Here's how the part is built. I have some questions about the finished solid (model axes, mm). A direction names the side the tool comes from. Coordinates: 2 decimals unless noted, no trailing zeros. Loops run counter-clockwise (first coordinate to the right, second up) from the corner with the lowest first, then second, coordinate; pieces in that order, holes last. Notation, with made-up numbers: (60.5, 31.25) -> (98.5, 31.25) arc R23 cw to (98.5, 47.25) -> close; hole circle Ø6 at (74, 73). An arc over 180 degrees is marked (long way). Answer as a JSON object with one key per item and string values. Group by question number.
Q1. I'm going to push flat-ended pins straight in: pin 1 (12 mm diameter, centred on x = -62.5, z = -59, fed in from +Y); pin 2 (3 mm diameter, centred on x = -132.25, y = 126.75, fed in from -Z); pin 3 (12 mm diameter, centred on x = -136, y = 125, fed in from +Z); pin 4 (3 mm diameter, centred on y = 130.5, z = -85.5, fed in from -X). Where does each tip first touch, or does it pass through?
Q2. I want a section at B-B on x = -138.75. Write out the boundary of the cut face in (y, z), then the cut area to 4 significant figures.
Q3. I want a section at D-D on z = -32.5. Write out the boundary of the cut face in (x, y).
Q4. Thinking about a two-plate mould opening in X: for faces 1 (the flat face through (-136, 128, -90)), 2 (the cylindrical face through (-62.2, 115.23, -90.14)), 3 (the flat face through (-50.5, 105, -62)), which applies, released by +X, released by -X, zero draft, split by the parting line, or undercut?
Q5. I want a section at A-A on y = 126.75. Write out the boundary of the cut face in (x, z).
Q6. I need wall thicknesses on line 1 (Y direction, x = -132, z = -94); line 2 (X direction, y = 135, z = -88.25); line 3 (Y direction, x = -58.5, z = -26). Which ranges of each line are inside material? Lowest first, please.
Q7. I want a section at C-C on x = -127. Write out the boundary of the cut face in (y, z), then the cut area to 3 significant figures.
Q8. On a 3-axis mill with a long thin cutter (end or side, diameter ignored), from which of +Z, -Z, +X, -X, +Y, -Y can I reach the whole of each face in a straight line? I mean faces 4 (the flat face through (-85, 128, -80)), 5 (the flat face through (-90, 145, -90)), 6 (the flat face through (-120.5, 128, -85)). Say none if no direction works.
Autodesk Inventor part; units mm, degrees
ref_plane "YZ Plane" through (0, 0, 0) normal (1, 0, 0) x (0, 1, 0)
ref_plane "XZ Plane" through (0, 0, 0) normal (0, 1, 0) x (-1, 0, 0)
ref_plane "XY Plane" through (0, 0, 0) normal (0, 0, 1) x (1, 0, 0)
sketch "Boceto2" plane through (0, 0, 0) normal (0, 1, 0) x (-1, 0, 0)
  line L0 (7.5, 100) -> (-7.5, 100)
  line L1 (-7.5, 100) -> (-7.5, -100)
  line L2 (-7.5, -100) -> (7.5, -100)
  line L3 (7.5, -100) -> (7.5, 100)
  line L4 (7.5, 100) -> (-7.5, -100) construction
  line L5 (-7.5, 100) -> (7.5, -100) construction
  point P0 (0, 0)
  dimension "d7" = 15
  dimension "d8" = 200
extrude "Extrusión1" add sketch "Boceto2" along normal blind 10
sketch "Boceto3" plane through (0, 10, 0) normal (0, 1, 0) x (1, 0, 0)
  circle A0 centre (3.25, 58.25) radius 1.75
  line L0 (5, 50) -> (-5, 50)
  line L1 (-5, 50) -> (-5, 60)
  line L2 (-5, 60) -> (5, 60)
  line L3 (5, 60) -> (5, 50)
  line L4 (5, 50) -> (-5, 60) construction
  line L5 (-5, 50) -> (5, 60) construction
  circle A1 centre (-3.25, 51.75) radius 1.75
  line L6 (7.5, 100) -> (-7.5, 100)
  line L7 (-7.5, 0) -> (3.408, 0)
  line L8 (5, -60) -> (5, -50)
  line L9 (-5, -60) -> (5, -60)
  line L10 (5, -50) -> (-5, -50)
  line L11 (-5, -50) -> (-5, -60)
  line L12 (-5, -50) -> (5, -60) construction
  circle A2 centre (-3.25, -51.75) radius 1.75
  line L13 (5, -50) -> (-5, -60) construction
  circle A3 centre (3.25, -58.25) radius 1.75
  line L14 (-7.5, -100) -> (7.5, -100)
  point P0 (0, 0)
  point P1 (-5, 55)
  point P2 (0, 100)
  point P3 (-5, -55)
  dimension "d11" = 3.5
  dimension "d12" = 1.75
  dimension "d13" = 1.75
  dimension "d14" = 1.75
  dimension "d15" = 1.75
  dimension "d16" = 10
  dimension "d17" = 10
  dimension "d19" = 40
  dimension "d81" = 40
hole "Agujero1" at (3.25, 10, 58.25) at (-3.25, 10, 51.75) at (3.25, 10, -58.25) at (-3.25, 10, -51.75) direction (0, -1, 0) diameter 3.5 end through all
sketch "Boceto4" plane through (0, 10, 0) normal (0, 1, 0) x (1, 0, 0)
  line L0 (-7.5, 100) -> (-7.5, -100)
  line L1 (-7.5, -100) -> (7.5, -100)
  line L2 (7.5, -100) -> (7.5, -80)
  line L3 (7.5, -80) -> (-7.5, -80)
  line L4 (-7.5, -80) -> (-7.5, -100)
  line L5 (-7.5, 0) -> (1.0116, 0)
  line L6 (-7.5, -100) -> (-7.5, 100)
  line L7 (-7.5, 100) -> (7.5, 100)
  line L8 (7.5, 100) -> (7.5, 80)
  line L9 (7.5, 80) -> (-7.5, 80)
  line L10 (-7.5, 80) -> (-7.5, 100)
  point P0 (0, 0)
  point P1 (-7.5, -80)
  point P2 (-7.5, 80)
  dimension "d27" = 15
  dimension "d28" = 20
extrude "Extrusión2" add sketch "Boceto4" along normal blind 80
sketch "Boceto5" plane through (0, 90, 0) normal (0, 1, 0) x (1, 0, 0)
  line L0 (-7.5, -100) -> (7.5, -100)
  line L1 (-7.5, -100) -> (49.5, -100)
  line L2 (49.5, -100) -> (49.5, 100)
  line L3 (49.5, 100) -> (-7.5, 100)
  line L4 (-7.5, 100) -> (-7.5, -100)
  line L5 (49.5, -100) -> (-150.5, -100)
  line L6 (-150.5, -100) -> (-150.5, 100)
  line L7 (-150.5, 100) -> (49.5, 100)
  line L8 (49.5, 100) -> (49.5, -100)
  point P0 (0, 0)
  point P1 (-7.5, 100)
  dimension "d31" = 57
  dimension "d32" = 200
  dimension "d75" = 200
extrude "Extrusión3" add sketch "Boceto5" along normal blind 110
sketch "Boceto6" plane through (0, 200, 0) normal (0, 1, 0) x (1, 0, 0)
  line L0 (49.5, 100) -> (7.5, 100)
  line L1 (49.5, 100) -> (29.5, 100)
  line L2 (29.5, 100) -> (29.5, 80)
  line L3 (7.5, -100) -> (49.5, -100)
  line L4 (28.5, -100) -> (28.5, -80)
  line L5 (-150.5, 100) -> (-150.5, -100)
  line L6 (29.5, 80) -> (-150.5, 80)
  line L7 (-150.5, 80) -> (-150.5, -80)
  line L8 (-150.5, -80) -> (29.5, -80)
  line L9 (29.5, -80) -> (29.5, 80)
  line L10 (-150.5, -100) -> (49.5, -100)
  point P0 (7.5, 80)
  point P1 (-50.5, -100)
  dimension "d36" = 20
  dimension "d37" = 20
  dimension "d38" = 20
  dimension "d77" = 20
extrude "Extrusión4" cut sketch "Boceto6" against normal blind 90 contours L8 L5 L6 L9
sketch "Boceto7" plane through (-150.5, 90, -100) normal (-1, 0, 0) x (0, 0, 1)
  line L0 (0, 110) -> (20, 110)
  line L1 (20, 110) -> (10, 110)
  line L2 (10, 110) -> (10, 20)
  line L3 (10, 20) -> (20, 20)
  line L4 (20, 20) -> (20, 110)
  line L5 (180, 110) -> (180, 20)
  line L6 (180, 110) -> (190, 110)
  line L7 (190, 110) -> (190, 20)
  line L8 (190, 20) -> (180, 20)
  line L9 (180, 20) -> (180, 110)
  line L10 (200, 0) -> (200, 110)
  line L11 (0, 0) -> (0, 110)
  line L12 (0, 110) -> (10, 110)
  line L13 (10, 110) -> (10, 20)
  line L14 (10, 20) -> (0, 20)
  line L15 (0, 20) -> (0, 110)
  line L16 (200, 110) -> (0, 110)
  line L17 (200, 110) -> (190, 110)
  line L18 (190, 110) -> (190, 20)
  line L19 (190, 20) -> (200, 20)
  line L20 (200, 20) -> (200, 110)
  point P0 (100, -90)
  dimension "d63" = 10
  dimension "d65" = 10
  dimension "d76" = 10
extrude "Extrusión5" cut sketch "Boceto7" against normal blind 30 contours L6 L7 L8 L5 | L0 L4 L3 L2
sketch "Boceto8" plane through (-7.5, 0, 100) normal (0, 0, 1) x (1, 0, 0)
  line L0 (-113, 110) -> (-113, 200)
  line L1 (-113, 200) -> (-113, 110)
  circle A0 centre (-124.75, 183.25) radius 1.75
  line L2 (-123, 175) -> (-133, 175)
  line L3 (-133, 175) -> (-133, 185)
  line L4 (-133, 185) -> (-123, 185)
  line L5 (-123, 185) -> (-123, 175)
  line L6 (-123, 175) -> (-133, 185) construction
  line L7 (-133, 175) -> (-123, 185) construction
  circle A1 centre (-131.25, 176.75) radius 1.75
  line L8 (-143, 200) -> (57, 200)
  line L9 (-143, 90) -> (-143, 200)
  line L10 (-113, 155) -> (-128, 155)
  line L11 (-123, 125) -> (-123, 135)
  line L12 (-133, 125) -> (-123, 125)
  line L13 (-123, 135) -> (-133, 125) construction
  line L14 (-123, 135) -> (-133, 135)
  line L15 (-133, 135) -> (-123, 125) construction
  circle A2 centre (-131.25, 133.25) radius 1.75
  line L16 (-133, 135) -> (-133, 125)
  circle A3 centre (-124.75, 126.75) radius 1.75
  line L17 (-143, 110) -> (-113, 110)
  point P0 (7.5, 0)
  point P1 (-133, 180)
  point P2 (-123, 180)
  point P3 (-133, 130)
  point P4 (-123, 130)
  dimension "d45" = 3.5
  dimension "d46" = 1.75
  dimension "d47" = 1.75
  dimension "d48" = 1.75
  dimension "d49" = 1.75
  dimension "d50" = 10
  dimension "d51" = 10
  dimension "d52" = 15
  dimension "d53" = 10
  dimension "d54" = 10
  dimension "d55" = 15
hole "Agujero2" at (-132.25, 183.25, 100) at (-138.75, 176.75, 100) at (-138.75, 133.25, 100) at (-132.25, 126.75, 100) direction (0, 0, -1) diameter 3.5 end through all
ref_plane "Plano de trabajo1" through (-150.5, 90, 100) normal (0, -1, 0) x (1, 0, 0)
split "Dividir1" plane through (-150.5, 90, 100) removes the side toward (0, -1, 0)
ref_plane "Plano de trabajo2" through (49.5, 90, 0) normal (0, 0, -1) x (-1, 0, 0)
ref_plane "Plano de trabajo3" through (-50.5, 90, 100) normal (1, 0, 0) x (0, 0, -1)
ref_plane "Plano de trabajo4" through (0, 145, 0) normal (0, 1, 0) x (1, 0, 0)
sketch "Boceto9" plane through (-150.5, 90, 100) normal (0, 0, 1) x (1, 0, 0)
  line L0 (85.0357, 30) -> (115.0357, 30)
  circle A0 centre (110.0357, 25) radius 1.75
  line L1 (90.0357, 25) -> (110.0357, 25)
  line L2 (115.0357, 30) -> (115.0357, 20)
  circle A1 centre (90.0357, 25) radius 1.75
  line L3 (85.0357, 20) -> (115.0357, 30) construction
  line L4 (85.0357, 30) -> (115.0357, 20) construction
  line L5 (85.0357, 20) -> (85.0357, 30)
  line L6 (115.0357, 20) -> (85.0357, 20)
  line L7 (200, 0) -> (200, 110)
  line L8 (200, 55) -> (88.2857, 55)
  circle A2 centre (90.0357, 85) radius 1.75
  line L9 (85.0357, 80) -> (115.0357, 80)
  line L10 (85.0357, 80) -> (115.0357, 90) construction
  line L11 (85.0357, 90) -> (85.0357, 80)
  line L12 (115.0357, 90) -> (85.0357, 90)
  line L13 (85.0357, 90) -> (115.0357, 80) construction
  circle A3 centre (110.0357, 85) radius 1.75
  line L14 (90.0357, 85) -> (110.0357, 85)
  line L15 (115.0357, 80) -> (115.0357, 90)
  line L16 (100.0357, 55) -> (185.099, 55) construction
  line L17 (160, 70) -> (160, 40)
  circle A4 centre (165, 45) radius 1.75
  line L18 (170, 40) -> (170, 70)
  line L19 (170, 70) -> (160, 40) construction
  line L20 (160, 40) -> (170, 40)
  line L21 (160, 70) -> (170, 40) construction
  circle A5 centre (165, 65) radius 1.75
  line L22 (165, 65) -> (165, 45)
  line L23 (170, 70) -> (160, 70)
  circle A6 centre (55, 65) radius 1.75
  line L24 (60, 70) -> (60, 40)
  line L25 (60, 40) -> (50, 40)
  circle A7 centre (55, 45) radius 1.75
  line L26 (55, 65) -> (55, 45)
  line L27 (60, 70) -> (50, 40) construction
  line L28 (50, 40) -> (50, 70)
  line L29 (50, 70) -> (60, 40) construction
  line L30 (50, 70) -> (60, 70)
  line L31 (30, 110) -> (30, 20)
  point P0 (150.5, -90)
  point P1 (100.0357, 34.7141)
  point P2 (100.0357, 34.7141)
  point P3 (85.0357, 36.6749)
  point P4 (115.0357, 25)
  point P5 (115.0357, 85)
  point P6 (189.1833, 40)
  point P7 (165, 70)
  point P8 (70.0357, 40)
  point P9 (55, 70)
  dimension "d89" = 10
  dimension "d90" = 30
  dimension "d91" = 5
  dimension "d92" = 5
  dimension "d93" = 5
  dimension "d94" = 5
  dimension "d95" = 30
  dimension "d96" = 5
  dimension "d97" = 5
  dimension "d98" = 3.5
  dimension "d99" = 5
  dimension "d100" = 5
  dimension "d101" = 5
  dimension "d102" = 5
  dimension "d103" = 5
  dimension "d104" = 20
hole "Agujero3" at (-60.4643, 175, 100) at (-40.4643, 175, 100) at (14.5, 155, 100) at (-95.5, 155, 100) at (-95.5, 135, 100) at (-60.4643, 115, 100) at (-40.4643, 115, 100) at (14.5, 135, 100) direction (0, 0, -1) diameter 3.5 end through all
sketch "Boceto10" plane through (49.5, 90, 100) normal (1, 0, 0) x (0, 0, -1)
  line L0 (85.0357, 30) -> (115.0357, 30)
  circle A0 centre (110.0357, 25) radius 1.75
  line L1 (90.0357, 25) -> (110.0357, 25)
  line L2 (115.0357, 30) -> (115.0357, 20)
  circle A1 centre (90.0357, 25) radius 1.75
  line L3 (85.0357, 30) -> (115.0357, 20) construction
  line L4 (85.0357, 20) -> (85.0357, 30)
  line L5 (115.0357, 20) -> (85.0357, 20)
  line L6 (85.0357, 20) -> (115.0357, 30) construction
  line L7 (160, 70) -> (160, 40)
  circle A2 centre (165, 45) radius 1.75
  line L8 (160, 40) -> (170, 40)
  line L9 (165, 65) -> (165, 45)
  circle A3 centre (165, 65) radius 1.75
  line L10 (170, 70) -> (160, 40) construction
  line L11 (170, 70) -> (160, 70)
  line L12 (160, 70) -> (170, 40) construction
  line L13 (170, 40) -> (170, 70)
  line L14 (40, 70) -> (40, 40)
  line L15 (35, 65) -> (35, 45)
  circle A4 centre (35, 65) radius 1.75
  line L16 (40, 40) -> (30, 40)
  line L17 (40, 70) -> (30, 40) construction
  line L18 (30, 70) -> (40, 40) construction
  line L19 (30, 70) -> (40, 70)
  line L20 (30, 40) -> (30, 70)
  circle A5 centre (35, 45) radius 1.75
  circle A6 centre (90.0357, 85) radius 1.75
  line L21 (85.0357, 80) -> (115.0357, 80)
  line L22 (115.0357, 80) -> (115.0357, 90)
  circle A7 centre (110.0357, 85) radius 1.75
  line L23 (90.0357, 85) -> (110.0357, 85)
  line L24 (85.0357, 80) -> (115.0357, 90) construction
  line L25 (85.0357, 90) -> (85.0357, 80)
  line L26 (115.0357, 90) -> (85.0357, 90)
  line L27 (85.0357, 90) -> (115.0357, 80) construction
  line L28 (0, 0) -> (0, 110)
  line L29 (200, 0) -> (200, 110)
  point P0 (100, -90)
  point P1 (100.0357, 34.7141)
  point P2 (100.0357, 34.7141)
  point P3 (85.0357, 36.6749)
  point P4 (115.0357, 25)
  point P5 (88.2857, 55)
  point P6 (189.1833, 40)
  point P7 (165, 70)
  point P8 (70.0357, 40)
  point P9 (35, 70)
  point P10 (115.0357, 85)
  point P11 (100.0357, 55)
  dimension "d112" = 10
  dimension "d113" = 30
  dimension "d114" = 5
  dimension "d115" = 5
  dimension "d116" = 5
  dimension "d117" = 5
  dimension "d118" = 5
  dimension "d119" = 5
  dimension "d120" = 3.5
  dimension "d121" = 5
  dimension "d122" = 5
  dimension "d123" = 5
  dimension "d124" = 5
  dimension "d125" = 5
  dimension "d126" = 30
  dimension "d127" = 30
hole "Agujero4" at (49.5, 175, 9.9643) at (49.5, 175, -10.0357) at (49.5, 155, 65) at (49.5, 135, 65) at (49.5, 115, 9.9643) at (49.5, 115, -10.0357) at (49.5, 135, -65) at (49.5, 155, -65) direction (-1, 0, 0) diameter 3.5 end through all
split "Dividir2" plane through (-50.5, 90, 100) removes the side toward (1, 0, 0)
split "Dividir3" plane through (0, 145, 0) removes the side toward (0, 1, 0)
split "Dividir4" plane through (49.5, 90, 0) removes the side toward (0, 0, 1)
properties part number "container_front_head_3"
Result set:
{
 "1": {"pin 1": "stops at y = 110", "pin 2": "passes through", "pin 3": "stops at z = -90", "pin 4": "stops at x = -120.5"},
 "2": {"outline": "(90, -100) -> (131.5, -100) -> (131.5, -90) -> (110, -90) -> (110, 0) -> (90, 0) -> close; (135, -100) -> (145, -100) -> (145, -90) -> (135, -90) -> close", "area": "2,315 mm²"},
 "3": {"outline": "(-150.5, 90) -> (-50.5, 90) -> (-50.5, 110) -> (-150.5, 110) -> close"},
 "4": {"face 1": "zero draft", "face 2": "undercut", "face 3": "released by +X"},
 "5": {"outline": "(-150.5, -100) -> (-134, -100) -> (-134, -90) -> (-150.5, -90) -> close; (-130.5, -100) -> (-50.5, -100) -> (-50.5, -80) -> (-120.5, -80) -> (-120.5, -90) -> (-130.5, -90) -> close"},
 "6": {"line 1": "y = 90 to 125.02, 128.48 to 145", "line 2": "x = -120.5 to -97.25, -93.75 to -50.5", "line 3": "y = 90 to 110"},
 "7": {"outline": "(90, -100) -> (145, -100) -> (145, -90) -> (110, -90) -> (110, 0) -> (90, 0) -> close", "area": "2,350 mm²"},
 "8": {"face 4": "+Z, +X, -X, +Y", "face 5": "+Z, -Z, +X, -X, +Y", "face 6": "+Z, -X, +Y"}
}
